```python
from build123d import *

# Parameters (mm, degrees)
SKETCH1_W           = 60
SKETCH1_H           = 90
BOSS_EXTRUDE1_DEPTH = 2
SKETCH2_W           = 60
SKETCH2_H           = 90
SKETCH2_W_2         = 56
SKETCH2_H_2         = 86
BOSS_EXTRUDE2_DEPTH = 10.6
CUT_EXTRUDE1_DEPTH  = 3
SKETCH15_W          = 90
SKETCH15_H          = 70
BOSS_EXTRUDE6_DEPTH = 2
BOSS_EXTRUDE7_DEPTH = 7.6
SKETCH4_R           = 0.9
BOSS_EXTRUDE3_DEPTH = 6
SKETCH18_W          = 2
SKETCH18_H          = 66
CUT_EXTRUDE11_DEPTH = 1.6
SKETCH7_W           = 14
SKETCH7_H           = 1
BOSS_EXTRUDE4_DEPTH = 2.6
SKETCH8_W           = 14
SKETCH8_H           = 2
CUT_EXTRUDE2_DEPTH  = 5
SKETCH9_W           = 15
SKETCH9_H           = 1
BOSS_EXTRUDE5_DEPTH = 7.6
SKETCH10_W          = 2
SKETCH10_H          = 7.7
CUT_EXTRUDE3_DEPTH  = 3.1
SKETCH11_W          = 2
SKETCH11_H          = 15.2
CUT_EXTRUDE4_DEPTH  = 1.22
SKETCH12_W          = 2
SKETCH12_H          = 12.76
CUT_EXTRUDE6_DEPTH  = 1.32
CUT_EXTRUDE7_REACH  = 157.202
FILLET6_R           = 1
CHAMFER2_SIZE       = 1.22
FILLET7_R           = 1
SKETCH19_W          = 88
SKETCH19_H          = 66
SKETCH19_W_2        = 86
SKETCH19_H_2        = 64
SKETCH19_R          = 0.9
BOSS_EXTRUDE9_DEPTH = 6
SKETCH20_W          = 4
SKETCH20_H          = 50.8
CUT_EXTRUDE12_DEPTH = 6
FILLET8_R           = 0.5
FILLET9_R           = 0.5
CUT_EXTRUDE13_DEPTH = 10


# Some blends are built 0.0001 mm under size
with BuildPart() as part:
    # Sketch1 → Boss-Extrude1 (new body)
    with BuildSketch(Plane(origin=(0, 0, 0), x_dir=(1, 0, 0), z_dir=(0, 1, 0))):
        Rectangle(SKETCH1_W, SKETCH1_H)
    extrude(amount=BOSS_EXTRUDE1_DEPTH)

    # Sketch2 → Boss-Extrude2 (add)
    with BuildSketch(Plane(origin=(0, 2, 0), x_dir=(1, 0, 0), z_dir=(0, 1, 0))):
        Rectangle(SKETCH2_W, SKETCH2_H)
        Rectangle(SKETCH2_W_2, SKETCH2_H_2, mode=Mode.SUBTRACT)
    extrude(amount=BOSS_EXTRUDE2_DEPTH)

    # Sketch3 → Cut-Extrude1 (cut)
    with BuildSketch(Plane(origin=(0, 12.6, 0), x_dir=(1, 0, 0), z_dir=(0, 1, 0))):
        Polygon((-28, -43), (28, -43), (28, 43), (-28, 43), (-28, 45), (30, 45), (30, -45), (-28, -45), align=None)
    extrude(amount=-CUT_EXTRUDE1_DEPTH, mode=Mode.SUBTRACT)

    # Sketch15 → Boss-Extrude6 (add)
    with BuildSketch(Plane.XZ):
        with Locations((75, -10)):
            Rectangle(SKETCH15_W, SKETCH15_H)
    extrude(amount=-BOSS_EXTRUDE6_DEPTH)

    # Sketch16 → Boss-Extrude7 (add)
    with BuildSketch(Plane(origin=(0, 2, 0), x_dir=(1, 0, 0), z_dir=(0, 1, 0))):
        Polygon((118, 43), (30, 43), (30, 45), (120, 45), (120, -25), (30, -25), (30, -23), (118, -23), align=None)
    extrude(amount=BOSS_EXTRUDE7_DEPTH)

    # Sketch4 → Boss-Extrude3 (add)
    # profile 1 of 5: a face of its own
    with BuildSketch(Plane(origin=(0, 2, 0), x_dir=(1, 0, 0), z_dir=(0, 1, 0))):
        with BuildLine():
            Line((24.2, -21.7), (27, -21.7))
            Line((27, -21.7), (27, -42))
            Line((27, -42), (-28, -42))
            Line((-28, -42), (-28, -43))
            Line((-28, -43), (28, -43))
            Line((28, -43), (28, 43))
            Line((28, 43), (5.8, 43))
            Line((5.8, 43), (5.8, 42))
            Line((5.8, 42), (19.4, 42))
            Line((19.4, 42), (27, 42))
            Line((27, 42), (27, 35.4))
            Line((27, 35.4), (27, -15.9))
            Line((27, -15.9), (24.2, -15.9))
            Line((24.2, -15.9), (24.2, -17.9))
            ThreePointArc((24.2, -17.9), (24.836396103, -18.163603897), (25.1, -18.8))
            ThreePointArc((25.1, -18.8), (24.836396103, -19.436396103), (24.2, -19.7))
            Line((24.2, -19.7), (24.2, -21.7))
        make_face()
    # profile 2 of 5: a face of its own
    with BuildSketch(Plane(origin=(0, 2, 0), x_dir=(1, 0, 0), z_dir=(0, 1, 0))):
        with BuildLine():
            Line((23.3, -21.7), (24.2, -21.7))
            Line((24.2, -21.7), (24.2, -19.7))
            ThreePointArc((24.2, -19.7), (23.3, -18.8), (24.2, -17.9))
            Line((24.2, -17.9), (24.2, -15.9))
            Line((24.2, -15.9), (23.3, -15.9))
            ThreePointArc((23.3, -15.9), (20.4, -18.8), (23.3, -21.7))
        make_face()
    # profile 3 of 5: a face of its own
    with BuildSketch(Plane(origin=(0, 2, 0), x_dir=(1, 0, 0), z_dir=(0, 1, 0))):
        with BuildLine():
            Line((-28, -15.9), (-28, -21.7))
            Line((-28, -21.7), (-24.5, -21.7))
            ThreePointArc((-24.5, -21.7), (-21.6, -18.8), (-24.5, -15.9))
            Line((-24.5, -15.9), (-28, -15.9))
        make_face()
        with Locations(Location((-24.8, -18.8, 0), (0, 0, 270))):
            Circle(SKETCH4_R, mode=Mode.SUBTRACT)
    # profile 4 of 5: a face of its own
    with BuildSketch(Plane(origin=(0, 2, 0), x_dir=(1, 0, 0), z_dir=(0, 1, 0))):
        with BuildLine():
            Line((-28, 43), (-28, 35.4))
            Line((-28, 35.4), (-24.6, 35.4))
            ThreePointArc((-24.6, 35.4), (-22.478679656, 36.278679656), (-21.6, 38.4))
            Line((-21.6, 38.4), (-21.6, 43))
            Line((-21.6, 43), (-28, 43))
        make_face()
        with Locations(Location((-24.8, 39.2, 0), (0, 0, 270))):
            Circle(SKETCH4_R, mode=Mode.SUBTRACT)
    # profile 5 of 5: a face of its own
    with BuildSketch(Plane(origin=(0, 2, 0), x_dir=(1, 0, 0), z_dir=(0, 1, 0))):
        with BuildLine():
            Line((22.4, 35.4), (27, 35.4))
            Line((27, 35.4), (27, 42))
            Line((27, 42), (19.4, 42))
            Line((19.4, 42), (19.4, 38.4))
            ThreePointArc((19.4, 38.4), (20.278679656, 36.278679656), (22.4, 35.4))
        make_face()
        with Locations(Location((24.2, 39.2, 0), (0, 0, 270))):
            Circle(SKETCH4_R, mode=Mode.SUBTRACT)
    extrude(amount=BOSS_EXTRUDE3_DEPTH)

    # Sketch18 → Cut-Extrude11 (cut)
    with BuildSketch(Plane(origin=(0, 9.6, 0), x_dir=(1, 0, 0), z_dir=(0, 1, 0))):
        with Locations((29, 10)):
            Rectangle(SKETCH18_W, SKETCH18_H)
    extrude(amount=-CUT_EXTRUDE11_DEPTH, mode=Mode.SUBTRACT)

    # Sketch7 → Boss-Extrude4 (add)
    with BuildSketch(Plane(origin=(0, 2, 0), x_dir=(1, 0, 0), z_dir=(0, 1, 0))):
        with Locations((-1.2, 42.5)):
            Rectangle(SKETCH7_W, SKETCH7_H)
    extrude(amount=BOSS_EXTRUDE4_DEPTH)

    # Sketch8 → Cut-Extrude2 (cut)
    with BuildSketch(Plane(origin=(0, 9.6, 0), x_dir=(1, 0, 0), z_dir=(0, 1, 0))):
        with Locations((-1.2, 44)):
            Rectangle(SKETCH8_W, SKETCH8_H)
    extrude(amount=-CUT_EXTRUDE2_DEPTH, mode=Mode.SUBTRACT)

    # Sketch9 → Boss-Extrude5 (add)
    with BuildSketch(Plane(origin=(0, 2, 0), x_dir=(1, 0, 0), z_dir=(0, 1, 0))):
        with Locations((-15.7, 42.5)):
            Rectangle(SKETCH9_W, SKETCH9_H)
    extrude(amount=BOSS_EXTRUDE5_DEPTH)

    # Sketch10 → Cut-Extrude3 (cut)
    with BuildSketch(Plane(origin=(0, 12.6, 0), x_dir=(1, 0, 0), z_dir=(0, 1, 0))):
        with Locations((-29, 32.32)):
            Rectangle(SKETCH10_W, SKETCH10_H)
    extrude(amount=-CUT_EXTRUDE3_DEPTH, mode=Mode.SUBTRACT)

    # Sketch11 → Cut-Extrude4 (cut)
    with BuildSketch(Plane(origin=(0, 12.6, 0), x_dir=(1, 0, 0), z_dir=(0, 1, 0))):
        with Locations((-29, 10.98)):
            Rectangle(SKETCH11_W, SKETCH11_H)
    extrude(amount=-CUT_EXTRUDE4_DEPTH, mode=Mode.SUBTRACT)

    # Sketch12 → Cut-Extrude6 (cut)
    with BuildSketch(Plane(origin=(0, 11.38, 0), x_dir=(1, 0, 0), z_dir=(0, 1, 0))):
        with Locations((-29, 10.98)):
            Rectangle(SKETCH12_W, SKETCH12_H)
    extrude(amount=-CUT_EXTRUDE6_DEPTH, mode=Mode.SUBTRACT)

    # Sketch13 → Cut-Extrude7 (cut, up to next)
    with BuildSketch(Plane(origin=(-28, 0, 0), x_dir=(0, 0, -1), z_dir=(1, 0, 0)), mode=Mode.PRIVATE) as cut_extrude7_sk1:
        with BuildLine():
            Line((-13.88, 12.6), (-7.48, 12.6))
            ThreePointArc((-7.48, 12.6), (-10.68, 9.4), (-13.88, 12.6))
        make_face()
    cut_extrude7_tool1 = extrude(cut_extrude7_sk1.sketch, amount=-CUT_EXTRUDE7_REACH, mode=Mode.PRIVATE) & part.part
    add(cut_extrude7_tool1.solids().sort_by_distance((-28, 11.241878, 10.68))[0], mode=Mode.SUBTRACT)

    # Fillet6
    fillet6_edges = [part.edges().sort_by_distance(p)[0] for p in [
        (-29, 11.38, -18.58),
        (-29, 11.38, -3.38),
    ]]
    fillet(fillet6_edges, radius=FILLET6_R)

    # Chamfer2
    chamfer2_edges = [part.edges().sort_by_distance(p)[0] for p in [
        (-29, 10.06, -17.36),
        (-29, 10.06, -4.6),
    ]]
    chamfer(chamfer2_edges, length=CHAMFER2_SIZE)

    # Fillet7
    # the kernel refuses this fillet: 1 mm, written as the material it adds along each edge
    with BuildSketch(Plane(origin=(-28, 10.06, -16.14), x_dir=(0, 0.7071067811865454, -0.7071067811865497), z_dir=(-1, 0, 0))) as fillet7_piece_1:
        with BuildLine():
            CenterArc((FILLET7_R * 0.414213562373, -FILLET7_R), FILLET7_R, 90, 45)
            Line((-FILLET7_R * 0.292893218813, -FILLET7_R * 0.292893218813), (0, 0))
            Line((0, 0), (FILLET7_R * 0.414213562373, 0))
        make_face()
    extrude(amount=2)
    with BuildSketch(Plane(origin=(-30, 10.06, -5.82), x_dir=(0, 0, -1), z_dir=(1, 0, 0))) as fillet7_piece_2:
        with BuildLine():
            CenterArc((FILLET7_R * 0.414213562373, FILLET7_R), FILLET7_R, 225, 45)
            Line((-FILLET7_R * 0.292893218813, FILLET7_R * 0.292893218813), (0, 0))
            Line((0, 0), (FILLET7_R * 0.414213562373, 0))
        make_face()
    extrude(amount=2)
    # the kernel refuses this fillet: 1 mm, written as the material it takes off along each edge
    with BuildSketch(Plane(origin=(-30.857621037, 11.38, -4.6), x_dir=(0, -1.0, 1.3882228699547056e-11), z_dir=(1, 0, 0)), Plane(origin=(-27.142378963, 11.38, -17.36), x_dir=(0, -1.0, -1.3891110483744069e-11), z_dir=(-1, 0, 0))) as fillet7_2_piece_1:
        with BuildLine():
            CenterArc((0.984822149, -0.465928927), FILLET7_R, 152.229642834, 20.707135911)
            Line((-0.007588926, -0.342964463), (-0.106830033, -0.330668017))
            ThreePointArc((-0.106830033, -0.330668017), (-0.1, -0.22), (-0.1, 0))
            Line((-0.1, 0), (0, 0.1))
            ThreePointArc((0, 0.1), (0.05, 0.1), (0.011517785, 0.046592893))
            Line((0.011517785, 0.046592893), (0.1, 0))
        make_face()
    extrude(amount=3.715242074, mode=Mode.SUBTRACT)

    # Sketch19 → Boss-Extrude9 (add)
    # profile 1 of 5: a face of its own
    with BuildSketch(Plane(origin=(0, 2, 0), x_dir=(1, 0, 0), z_dir=(0, 1, 0))):
        with Locations((74, 10)):
            Rectangle(SKETCH19_W, SKETCH19_H)
        with Locations((74, 10)):
            Rectangle(SKETCH19_W_2, SKETCH19_H_2, mode=Mode.SUBTRACT)
    # profile 2 of 5: a face of its own
    with BuildSketch(Plane(origin=(0, 2, 0), x_dir=(1, 0, 0), z_dir=(0, 1, 0))):
        with BuildLine():
            Line((37.6, 38.4), (37.6, 42))
            Line((37.6, 42), (31, 42))
            Line((31, 42), (31, 35.4))
            Line((31, 35.4), (34.6, 35.4))
            ThreePointArc((34.6, 35.4), (36.721320344, 36.278679656), (37.6, 38.4))
        make_face()
        with Locations(Location((33.8, 39.200675532, 0), (0, 0, 270))):
            Circle(SKETCH19_R, mode=Mode.SUBTRACT)
    # profile 3 of 5: a face of its own
    with BuildSketch(Plane(origin=(0, 2, 0), x_dir=(1, 0, 0), z_dir=(0, 1, 0))):
        with BuildLine():
            Line((117, 35.4), (117, 42))
            Line((117, 42), (110.4, 42))
            Line((110.4, 42), (110.4, 38.4))
            ThreePointArc((110.4, 38.4), (111.278679656, 36.278679656), (113.4, 35.4))
            Line((113.4, 35.4), (117, 35.4))
        make_face()
        with Locations(Location((114.2, 39.200675532, 0), (0, 0, 270))):
            Circle(SKETCH19_R, mode=Mode.SUBTRACT)
    # profile 4 of 5: a face of its own
    with BuildSketch(Plane(origin=(0, 2, 0), x_dir=(1, 0, 0), z_dir=(0, 1, 0))):
        with BuildLine():
            Line((117, -22), (117, -15.4))
            Line((117, -15.4), (113.4, -15.4))
            ThreePointArc((113.4, -15.4), (111.278679656, -16.278679656), (110.4, -18.4))
            Line((110.4, -18.4), (110.4, -22))
            Line((110.4, -22), (117, -22))
        make_face()
        with Locations(Location((114.2, -18.58, 0), (0, 0, 270))):
            Circle(SKETCH19_R, mode=Mode.SUBTRACT)
    # profile 5 of 5: a face of its own
    with BuildSketch(Plane(origin=(0, 2, 0), x_dir=(1, 0, 0), z_dir=(0, 1, 0))):
        with BuildLine():
            Line((34.6, -15.4), (31, -15.4))
            Line((31, -15.4), (31, -22))
            Line((31, -22), (37.6, -22))
            Line((37.6, -22), (37.6, -18.4))
            ThreePointArc((37.6, -18.4), (36.721320344, -16.278679656), (34.6, -15.4))
        make_face()
        with Locations(Location((33.8, -18.58, 0), (0, 0, 270))):
            Circle(SKETCH19_R, mode=Mode.SUBTRACT)
    extrude(amount=BOSS_EXTRUDE9_DEPTH)

    # Sketch20 → Cut-Extrude12 (cut)
    with BuildSketch(Plane(origin=(0, 8, 0), x_dir=(1, 0, 0), z_dir=(0, 1, 0))):
        with Locations((29, 10)):
            Rectangle(SKETCH20_W, SKETCH20_H)
    extrude(amount=-CUT_EXTRUDE12_DEPTH, mode=Mode.SUBTRACT)

    # Fillet8
    fillet8_edges = [part.edges().sort_by_distance(p)[0] for p in [
        (27, 5, 15.9),
    ]]
    fillet(fillet8_edges, radius=FILLET8_R - 0.0001)  # a hair under: the kernel refuses the full size

    # Fillet9
    fillet9_edges = [part.edges().sort_by_distance(p)[0] for p in [
        (27, 5, 15.4),
    ]]
    fillet(fillet9_edges, radius=FILLET9_R)

    # Sketch21 → Cut-Extrude13 (cut)
    with BuildSketch(Plane(origin=(0, 0, -45), x_dir=(-1, 0, 0), z_dir=(0, 0, -1))):
        with BuildLine():
            Line((-110, 9.6), (-100, 9.6))
            ThreePointArc((-100, 9.6), (-105, 4.6), (-110, 9.6))
        make_face()
    extrude(amount=-CUT_EXTRUDE13_DEPTH, mode=Mode.SUBTRACT)


solid = part.part
```
Input: part model. Units: mm. Frame: model coordinates. A direction names the side the tool comes from. Coordinates: 2 decimals unless noted, no trailing zeros. Loops run counter-clockwise (first coordinate to the right, second up) from the corner with the lowest first, then second, coordinate; pieces in that order, holes last. Notation, with made-up numbers: M 59.5,-33.5 L 104.5,-33.5 A33 ccw 104.5,-5.5 Z; hole C -26.75,-19.75 d4. An arc over 180 degrees is marked long. Use a Markdown table: item, result. Add a question column.
1) Section A-A, the plane x = 108. Return the cut outline in (y, z).
2) Section C-C, the plane x = 89.5. Return the cut outline in (y, z).
3) Draft query along X for faces 4 (the flat face through (-1, 4.6, -44)), 5 (the cylindrical face through (36.74, 4.96, 16.3)), 6 (the flat face through (-30, 6, -1)), 7 (the flat face through (44, 5, -45)). Return one class per face: +X half, -X half, draft (parallel to the pull), parting line (faces both ways), or undercut.
4) Set-up query: faces 1 (the flat face through (5.8, 7, -44)), 2 (the flat face through (37.6, 5, -40)), 3 (the cylindrical face through (-29, 9.4, 10.6)). Return all of +Z, -Z, +X, -X, +Y, -Y with unobstructed straight access to the full face (end or side cutting, diameter ignored); none if empty.
5) Pin query (flat end, axial travel): P1, Ø2, axis at x = -8.5, z = -16.5, coming from the +Y side; P2, Ø2, axis at x = 24.5, z = -39, coming from the +Y side; P3, Ø1.3, axis at x = 65, y = 8.5, coming from the +Z side. Return the tip coordinate at first contact, or that it passes through.
6) Section B-B, the plane z = 3. Return the cut outline in (x, y), plus the area to 3 significant figures.
7) Line query: L1, parallel to Z at x = 33.8, y = 4.1; L2, parallel to Z at x = 69.5, y = 9.25; L3, parallel to X at y = 9.25, z = 20. Output: solid intervals per line, ascending. Write a range as from..to.
Answer below:
| question | item | result |
|---|---|---|
| 1 | outline | M 0,-45 L 5.6,-45 L 5.6,-42 L 2,-42 L 2,22 L 8,22 L 8,23 L 9.6,23 L 9.6,25 L 0,25 Z |
| 2 | outline | M 0,-45 L 9.6,-45 L 9.6,-43 L 8,-43 L 8,-42 L 2,-42 L 2,22 L 8,22 L 8,23 L 9.6,23 L 9.6,25 L 0,25 Z |
| 3 | face 4 | undercut |
| 3 | face 5 | undercut |
| 3 | face 6 | -X half |
| 3 | face 7 | draft |
| 4 | face 1 | -Z, +Y |
| 4 | face 2 | +Y |
| 4 | face 3 | -X, +Y |
| 5 | P1 | y = 2 |
| 5 | P2 | y = 8 |
| 5 | P3 | z = 25 |
| 6 | outline | M -30,0 L 120,0 L 120,9.6 L 118,9.6 L 118,8 L 117,8 L 117,2 L -28,2 L -28,12.6 L -30,12.6 Z |
| 6 | area | 342 mm2 |
| 7 | L1 | -45..-40.1, -38.3..-35.4, 15.4..17.68, 19.48..25 |
| 7 | L2 | -45..-43, 23..25 |
| 7 | L3 | -30..-28, 118..120 |
